Here's the drawing with two shaded views (mm, measured from the low corner). I have some questions. A direction names the side the tool comes from. Give positions to 0.01 mm unless a question says otherwise; leave off trailing zeros. Loops run counter-clockwise (first coordinate to the right, second up) from the corner with the lowest first, then second, coordinate; pieces in that order, holes last. Notation, with made-up numbers: M 45,73.5 L 71,73.5 A19 cw 71,81.5 Z; hole C -16.75,35 d10. An arc over 180 degrees is marked long. Put each result on its own line as item: value. Start each with the question number.
1) Imagine slicing it at D-D (x = 6). Write out the boundary of the cut face in (y, z).
2) If we mould it in two halves opening along X, with no side actions, what happens to the marked faces 5, 6, 7 and 8? For each: +X half, -X half, draft (parallel to the pull), parting line (faces both ways), or undercut.
3) Imagine slicing it at C-C (y = 11.5). Write out the boundary of the cut face in (x, z) (1 decimal).
4) Imagine slicing it at B-B (z = 7.5). Write out the boundary of the cut face in (x, y), then the cut area to 3 significant figures.
5) Please list where these lines run through material, in increasing order: line 1 along Z through (x, y) = (3, 19.5); line 2 along X through (y, z) = (7, 9.5); line 3 along Z through (x, y) = (16, 16.75) (1 decimal). Write a range as from..to.
6) For P1, Ø12, axis at x = 15, y = 18, coming from the +Z side; P2, Ø3.5, axis at x = 9, y = 7, coming from the -Z side; P3, Ø1, axis at x = 21.5, z = 37, coming from the -Y side (1 decimal); P4, Ø2.5, axis at y = 6.5, z = 8, coming from the +X side, each with a flat end and sliding along its axis, tell me the tip position at first contact or that it passes through.
7) Imagine slicing it at A-A (x = 3.25). Write out the boundary of the cut face in (y, z).
8) For the marked faces 1, 2, 3 and 4, which set-ups out of +Z, -Z, +X, -X, +Y, -Y let a thin tool reach every point of the face, with its end or its side?
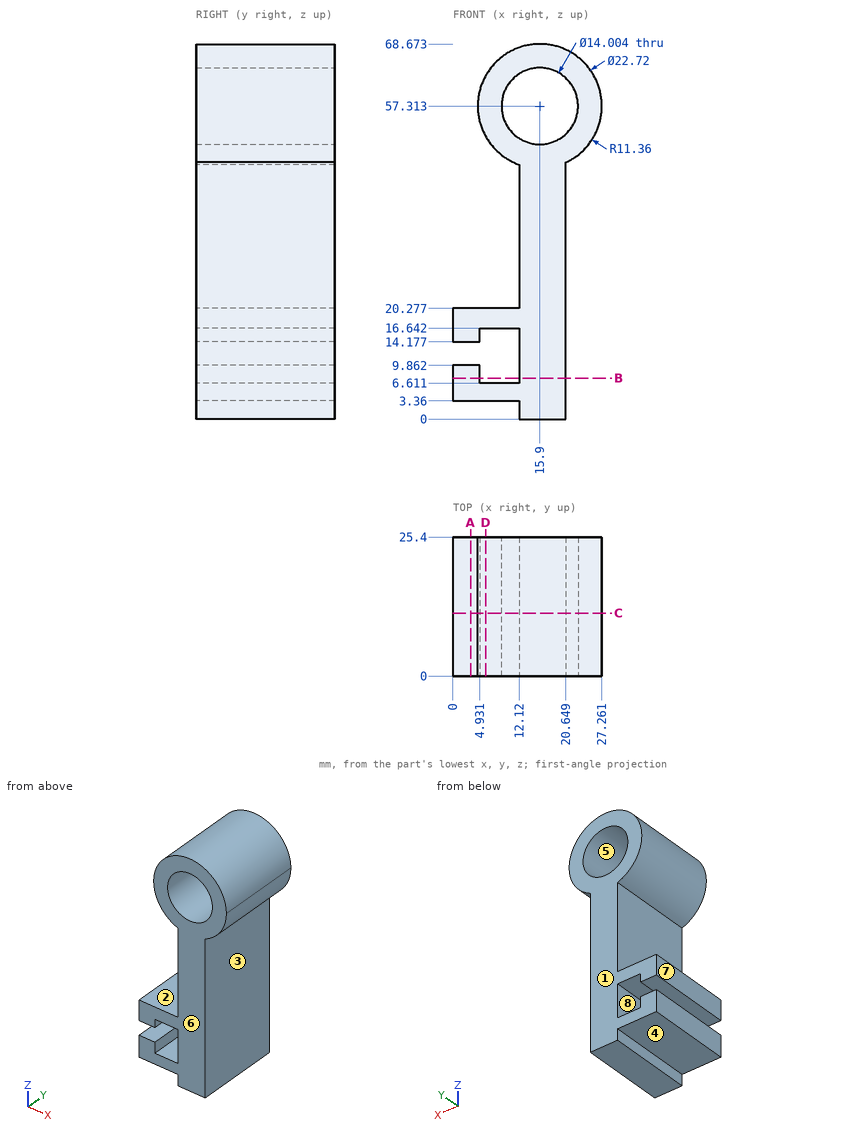
Recorded:
1. outline: M 0,3.36 L 25.4,3.36 L 25.4,6.61 L 0,6.61 Z; M 0,16.64 L 25.4,16.64 L 25.4,20.28 L 0,20.28 Z; M 0,51.74 L 25.4,51.74 L 25.4,62.88 L 0,62.88 Z
2. face 5: undercut
2. face 6: draft
2. face 7: -X half
2. face 8: undercut
3. outline: M 0,3.4 L 12.1,3.4 L 12.1,0 L 20.6,0 L 20.6,47 A11.4 ccw 27.3,57.3 A11.4 ccw long 12.1,46.6 L 12.1,20.3 L 0,20.3 L 0,14.2 L 4.9,14.2 L 4.9,16.6 L 12.1,16.6 L 12.1,6.6 L 4.9,6.6 L 4.9,9.9 L 0,9.9 Z; hole C 15.9,57.3 d14
4. outline: M 0,0 L 4.93,0 L 4.93,25.4 L 0,25.4 Z; M 12.12,0 L 20.65,0 L 20.65,25.4 L 12.12,25.4 Z
4. area: 342 mm²
5. line 1: 3.36..9.86, 14.18..20.28
5. line 2: 0..4.93, 12.12..20.65
5. line 3: 0..50.3, 64.3..68.7
6. P1: z = 68.67
6. P2: z = 3.36
6. P3: through
6. P4: x = 20.65
7. outline: M 0,3.36 L 25.4,3.36 L 25.4,9.86 L 0,9.86 Z; M 0,14.18 L 25.4,14.18 L 25.4,20.28 L 0,20.28 Z
8. face 1: +Z, -Z, +X, -X, +Y
8. face 2: -X, +Y, -Y
8. face 3: -Z, +X, +Y, -Y
8. face 4: -Z, -X, +Y, -Y
